Autodesk Inventor part; units mm, degrees
ref_plane "Work Plane7" through (0, 79.375, 0) normal (0, 1, 0) x (-1, 0, 0)
ref_plane "YZ Plane" through (0, 0, 0) normal (1, 0, 0) x (0, 1, 0)
ref_plane "XY Plane" through (0, 0, 0) normal (0, 0, 1) x (1, 0, 0)
sketch "Sketch8" plane through (0, 0, 0) normal (0, 0, 1) x (1, 0, 0)
  arc A0 (76.1338, 3.175) -> (-76.1338, 3.175) centre (0, 0) ccw
  arc A1 (81.9986, 9.525) -> (-81.9986, 9.525) centre (0, 0) ccw
  line L0 (-82.4889, 3.175) -> (-101.5389, 3.175)
  line L1 (-101.5389, 3.175) -> (-101.5389, 9.525)
  line L2 (-101.5389, 9.525) -> (-81.9986, 9.525)
  line L3 (0, 0) -> (0, 82.55) construction
  line L4 (-82.4889, 3.175) -> (-76.1338, 3.175)
  line L5 (82.4889, 3.175) -> (101.5389, 3.175)
  line L6 (101.5389, 3.175) -> (101.5389, 9.525)
  line L7 (101.5389, 9.525) -> (81.9986, 9.525)
  line L8 (82.4889, 3.175) -> (76.1338, 3.175)
  dimension "d52" = 152.4
  dimension "d53" = 6.35
  dimension "d54" = 19.05
  dimension "d55" = 3.175
  dimension "d56" = 6.35
extrude "Extrusion5" add sketch "Sketch8" along normal mid plane 76.2
sketch "Sketch9" plane through (-101.5389, 9.525, 38.1) normal (0, 1, 0) x (1, 0, 0)
  line L0 (19.5403, 0) -> (0, 0) construction
  line L1 (9.7701, 0) -> (9.7701, 76.2) construction
  line L2 (25.4051, 76.2) -> (0, 76.2) construction
  line L3 (9.7701, 25.4) -> (9.7701, 101.6) construction
  line L4 (9.7701, 50.8) -> (9.7701, 127) construction
  point P0 (101.5389, 38.1)
  point P1 (9.7701, 12.7)
  point P2 (9.7701, 38.1)
  point P3 (9.7701, 63.5)
  dimension "d59" = 12.7
  dimension "d62" = 25.4
hole "Hole3" at (-91.7688, 9.525, 25.4) at (-91.7688, 9.525, 0) at (-91.7688, 9.525, -25.4) direction (0, -1, 0) diameter 6.7564 end through all
mirror "Mirror3" about plane through (0, 0, 0) normal (1, 0, 0) of "Hole3"
ref_plane "Work Plane7" through (0, 79.375, 0) normal (0, 1, 0) x (-1, 0, 0)
sketch "Sketch20" plane through (0, 79.375, 0) normal (0, 1, 0) x (-1, 0, 0)
  circle A0 centre (0, 0) radius 12.7
  dimension "d101" = 25.4
extrude "Extrusion11" add sketch "Sketch20" along normal blind 50.8
sketch "Sketch22" plane through (0, 130.175, 0) normal (0, 1, 0) x (1, 0, 0)
  circle A0 centre (0, 0) radius 6.35
  dimension "d111" = 12.7
extrude "Extrusion13" cut sketch "Sketch22" against normal blind 25.4
properties part number "tubeBracketV02" material "ABS Plastic"
The model under review builds one solid part; all positions refer to its coordinate system, in mm. A direction names the side the tool comes from. Coordinates: 2 decimals unless noted, no trailing zeros. Order: outer loops, then holes, each group sorted by start corner. A loop starts at its lowest first (then second) coordinate and runs counter-clockwise, first axis right, second up. Notation, with made-up numbers: (4, 51.5) -> (29, 51.5) arc R8 cw to (29, 55.5) -> close; hole circle Ø10 at (43.5, -33). An arc over 180 degrees is marked (long way). Answer in a Markdown table with one row per item.
(1) Wall thickness on line 1 along Z through (x, y) = (0, 124.25); line 2 along X through (y, z) = (6.75, 25.4); line 3 along X through (y, z) = (5, 0): over which ranges is each line inside the solid? List them lowest first.
Answers:
| item | result |
|---|---|
| line 1 | -12.7 to -6.35, 6.35 to 12.7 |
| line 2 | -101.54 to -95.15, -88.39 to -75.9, 75.9 to 88.39, 95.15 to 101.54 |
| line 3 | -101.54 to -95.15, -88.39 to -76.04, 76.04 to 88.39, 95.15 to 101.54 |
(2) Consider section B-B (y = 23). Write out the cut boundary in (x, z).
Answers:
| item | result |
|---|---|
| outline | (-79.28, -38.1) -> (-72.65, -38.1) -> (-72.65, 38.1) -> (-79.28, 38.1) -> close; (72.65, -38.1) -> (79.28, -38.1) -> (79.28, 38.1) -> (72.65, 38.1) -> close |
(3) Machinability: for faces 5 (the flat face through (-96, 9.525, -1)), 6 (the cylindrical face through (-1.38, 117.65, 6.2)), 7 (the cylindrical face through (-88.772, 6.306, 1.559)), 8 (the flat face through (86, 3.175, -1)), 9 (the flat face through (96, 9.525, -1)), which of the approach directions +Z, -Z, +X, -X, +Y, -Y give a long, thin tool a straight path to every point of the face, cutting with its end or side? Answer none if there is none.
Answers:
| item | result |
|---|---|
| face 5 | +Z, -Z, -X, +Y |
| face 6 | +Y |
| face 7 | +Y, -Y |
| face 8 | +Z, -Z, +X, -X, -Y |
| face 9 | +Z, -Z, +X, +Y |
(4) The part is to be moulded in two halves that separate along Z. For faces 1 (the flat face through (-101.539, 6, -1)), 2 (the flat face through (-16, 75, -38.1)), 3 (the flat face through (0, 104.775, 0)), 4 (the cylindrical face through (-6.827, 105.53, -10.709)), say which applies: +Z half, -Z half, draft (parallel to the pull), parting line (faces both ways), or undercut.
Answers:
| item | result |
|---|---|
| face 1 | draft |
| face 2 | -Z half |
| face 3 | undercut |
| face 4 | parting line |
(5) Consider section D-D (z = 0). Write out the cut boundary in (x, y) (3 decimals).
Answers:
| item | result |
|---|---|
| outline | (-101.539, 3.175) -> (-95.147, 3.175) -> (-95.147, 9.525) -> (-101.539, 9.525) -> close; (-88.391, 3.175) -> (-76.134, 3.175) arc R76.2 cw to (76.134, 3.175) -> (88.391, 3.175) -> (88.391, 9.525) -> (81.999, 9.525) arc R82.55 ccw to (12.7, 81.567) -> (12.7, 130.175) -> (6.35, 130.175) -> (6.35, 104.775) -> (-6.35, 104.775) -> (-6.35, 130.175) -> (-12.7, 130.175) -> (-12.7, 81.567) arc R82.55 ccw to (-81.999, 9.525) -> (-88.391, 9.525) -> close; (95.147, 3.175) -> (101.539, 3.175) -> (101.539, 9.525) -> (95.147, 9.525) -> close |
(6) Consider section A-A (z = 25.4). Write out the cut boundary in (x, y) (3 decimals).
Answers:
| item | result |
|---|---|
| outline | (-101.539, 3.175) -> (-95.147, 3.175) -> (-95.147, 9.525) -> (-101.539, 9.525) -> close; (-88.391, 3.175) -> (-76.134, 3.175) arc R76.2 cw to (76.134, 3.175) -> (88.391, 3.175) -> (88.391, 9.525) -> (81.999, 9.525) arc R82.55 ccw to (-81.999, 9.525) -> (-88.391, 9.525) -> close; (95.147, 3.175) -> (101.539, 3.175) -> (101.539, 9.525) -> (95.147, 9.525) -> close |
(7) Consider section C-C (x = 0). Write out the cut boundary in (y, z) (3 decimals).
Answers:
| item | result |
|---|---|
| outline | (76.2, -38.1) -> (82.55, -38.1) -> (82.55, -12.7) -> (130.175, -12.7) -> (130.175, -6.35) -> (104.775, -6.35) -> (104.775, 6.35) -> (130.175, 6.35) -> (130.175, 12.7) -> (82.55, 12.7) -> (82.55, 38.1) -> (76.2, 38.1) -> close |
(8) Insertion check: pin 1 (8 mm diameter, centred on x = -91.77, z = -25.4, fed in from +Y) (3 decimals); pin 2 (6 mm diameter, centred on x = 45.5, z = 16.5, fed in from +Y); pin 3 (6.5 mm diameter, centred on x = 0, z = 1.5, fed in from +Y) (3 decimals). Each pin has a flat end and moves straight along its axis. Give the tip position at first contact, or say it passes through.
Answers:
| item | result |
|---|---|
| pin 1 | y = 9.525 |
| pin 2 | y = 70.77 |
| pin 3 | y = 104.775 |
